Autodesk Inventor part; units mm, degrees
ref_plane "YZ Plane" through (0, 0, 0) normal (1, 0, 0) x (0, 1, 0)
ref_plane "XZ Plane" through (0, 0, 0) normal (0, 1, 0) x (-1, 0, 0)
ref_plane "XY Plane" through (0, 0, 0) normal (0, 0, 1) x (1, 0, 0)
sketch "草圖1" plane through (0, 0, 0) normal (0, 1, 0) x (-1, 0, 0)
  circle A0 centre (0, 0) radius 47.5
  dimension "d0" = 95
extrude "擠出1" add sketch "草圖1" along normal blind 3
sketch "草圖2" plane through (0, 0, 0) normal (1, 0, 0) x (0, 1, 0)
  line L0 (3, -47.5) -> (3, 47.5)
  line L1 (0, -47.5) -> (0, 47.5)
  line L2 (64.2836, 18.923) -> (61.7124, 21.9872)
  line L3 (61.7124, 21.9872) -> (0.4288, -29.4358)
  line L4 (0.4288, -29.4358) -> (3, -32.5)
  line L5 (3, -32.5) -> (64.2836, 18.923)
  point P0 (0, 0)
  dimension "d3" = 4
  dimension "d4" = 80
  dimension "d5" = 50
  dimension "d6" = 15
extrude "擠出2" add sketch "草圖2" along normal mid plane 10
sketch "草圖3" plane through (5, 64.2836, 18.923) normal (0, 0.6428, -0.766) x (-1, 0, 0)
  line L0 (10, 0) -> (0, 0)
  line L1 (0, -80) -> (0, 0)
  line L2 (10, -80) -> (0, -80)
  line L3 (10, 0) -> (10, -80)
  circle A0 centre (5, -10) radius 1.5
  circle A1 centre (5, -55) radius 1.5
  point P0 (5, -61.4075)
  dimension "d9" = 3
  dimension "d10" = 3
  dimension "d11" = 45
  dimension "d15" = 10
extrude "擠出3" cut sketch "草圖3" against normal blind 10 contours A0 | A1
properties part number "CB_middle_v1"
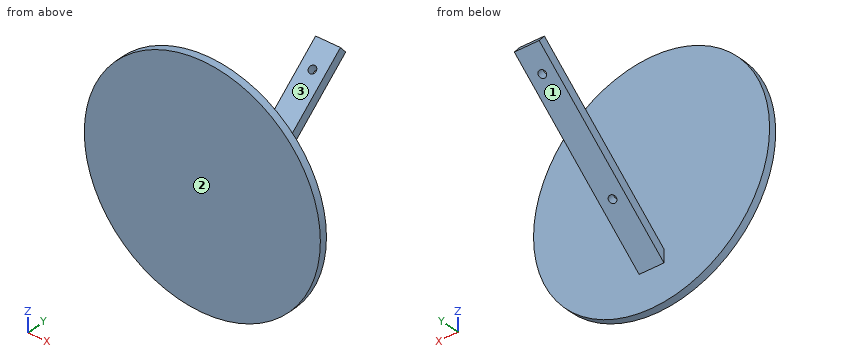
The model under review builds one solid part; all positions refer to its coordinate system, in mm. Face numbers are marked on the shaded views. Coordinates: 2 decimals unless noted, no trailing zeros. Write each loop counter-clockwise with the first axis right and the second up, starting at its lowest first coordinate (ties: lowest second). Pieces come first, ordered by that corner, then holes. Notation, with made-up numbers: (-31, 34.25) -> (-10, 34.25) arc R22 cw to (-10, 72.25) -> close; hole circle Ø11 at (-27.75, 46). An arc over 180 degrees is marked (long way). Answer in a Markdown table with one row per item.
1. Wall thickness on probe 1 along Y at (x, z) = (3.5, -42); probe 2 along Y at (x, z) = (2, -11.5); probe 3 along Y at (x, z) = (-2, 7): over which ranges is each line inside the solid? List them lowest first. Write a range as [from, to].
Answers below:
| item | result |
|---|---|
| probe 1 | y = [0, 3] |
| probe 2 | y = [0, 3], [21.8, 28.03] |
| probe 3 | y = [0, 3], [43.85, 50.07] |
2. We need section D-D, the plane x = -13.5. State the section outline as (y, z) points, and give its area (3 significant figures).
Answers below:
| item | result |
|---|---|
| outline | (0, -45.54) -> (3, -45.54) -> (3, 45.54) -> (0, 45.54) -> close |
| area | 273 mm^2 |
3. Clearance check with flat-ended pins moving along their axes: pin 1 Ø16.5 at (y, z) = (29.5, -12.5) entering from +X; pin 2 Ø1.5 at (x, y) = (2.5, 15) entering from +Z; pin 3 Ø1 at (x, z) = (31, 11) entering from +Y; pin 4 Ø2 at (y, z) = (26, -6) entering from -X. State where each tip first meets the part, or that it passes through.
Answers below:
| item | result |
|---|---|
| pin 1 | stops at x = 5 |
| pin 2 | stops at z = -16.58 |
| pin 3 | stops at y = 3 |
| pin 4 | passes through |
4. We need section B-B, the plane x = 0. State the section outline as (y, z) points, and give its area (3 significant figures).
Answers below:
| item | result |
|---|---|
| outline | (0, -47.5) -> (3, -47.5) -> (3, -32.5) -> (21, -17.39) -> (18.43, -14.33) -> (3, -27.28) -> (3, 47.5) -> (0, 47.5) -> close; (20.73, -12.4) -> (23.3, -15.47) -> (55.47, 11.53) -> (52.9, 14.6) -> close; (55.2, 16.52) -> (57.77, 13.46) -> (64.28, 18.92) -> (61.71, 21.99) -> close |
| area | 574 mm^2 |
5. We need section A-A, the plane z = 3. State the section outline as (x, y) points, and give its area (3 significant figures).
Answers below:
| item | result |
|---|---|
| outline | (-47.41, 0) -> (47.41, 0) -> (47.41, 3) -> (-47.41, 3) -> close; (-5, 39.08) -> (5, 39.08) -> (5, 45.31) -> (-5, 45.31) -> close |
| area | 347 mm^2 |
6. Draft analysis for pull direction Y (two halves, no side actions). For the marked faces 1, 2 and 3, state which applies: +Y half, -Y half, draft (parallel to the pull), parting line (faces both ways), or undercut.
Answers below:
| item | result |
|---|---|
| face 1 | +Y half |
| face 2 | -Y half |
| face 3 | undercut |
7. We need section C-C, the plane y = 33. State the section outline as (x, z) points, and give its area (3 significant figures).
Answers below:
| item | result |
|---|---|
| outline | (-5, -7.33) -> (5, -7.33) -> (5, -2.11) -> (-5, -2.11) -> close |
| area | 52.2 mm^2 |
